For this review, take the finished solid that the model builds, in its own axes (mm). A direction names the side the tool comes from. Give positions to 0.01 mm unless a question says otherwise; leave off trailing zeros. Write each loop counter-clockwise with the first axis right and the second up, starting at its lowest first coordinate (ties: lowest second). Pieces come first, ordered by that corner, then holes.
Q1. Machinability: for faces 1 (the flat face through (-3.175, -3, -16)), 2 (the cylindrical face through (0.2, -3.1, 25.4)), which of the approach directions +Z, -Z, +X, -X, +Y, -Y give a long, thin tool a straight path to every point of the face, cutting with its end or side? Answer none if there is none.
Q2. We need section B-B (y = -1.5). Write out the cut boundary in (x, z) (3 decimals).
Q3. We need section C-C (z = -16.5). Write out the cut boundary in (x, y) (3 decimals), then the cut area to 3 significant figures.
Q4. Insertion check: P1, Ø3, axis at y = -4.5, z = -16.5, coming from the +X side; P2, Ø3, axis at y = -4.5, z = -16, coming from the -X side; P3, Ø1.5, axis at x = -21.5, y = -3.5, coming from the -Z side. Each pin has a flat end and moves straight along its axis. Give the tip position at first contact, or say it passes through.
Q5. Mouldability with a two-part tool opening along Z and no side actions: class faces 3 (the cylindrical face through (-19.212, -3.131, 11.173)), 4 (the flat face through (0, -3, -25.4)), 5 (the flat face through (-21.867, -3.131, 12.925)), 6 (the flat face through (7, -6.35, 2)) as released by +Z, released by -Z, zero draft, split by the parting line, or undercut.
Q6. We need section A-A (x = 0). Write out the cut boundary in (y, z) (3 decimals), then the cut area to 3 significant figures.
Q7. For line 1 (Z direction, x = 0, y = -2.5) (3 decimals); line 2 (X direction, y = -1.25, z = 9); line 3 (X direction, y = -4.5, z = 5), list the stretches that pass through material, from the lowest coordinate up.
Q8. We need section D-D (z = 0). Write out the cut boundary in (x, y), then the cut area to 3 significant figures.
```python
from build123d import *

# Parameters (mm, degrees)
F0_R     = 6.35
F1_DEPTH = 6.35
F3_DEPTH = 25.4


with BuildPart() as f1:
    # F0 (on Front) → F1 (new body)
    with BuildSketch(Plane.XZ):
        with BuildLine():
            Line((-18.594091, -25.4), (18.594091, -25.4))
            ThreePointArc((18.594091, -25.4), (21.997045, -12.7), (31.294091, -3.402955))
            Line((31.294091, -3.402955), (12.7, 28.802955))
            ThreePointArc((12.7, 28.802955), (0, 25.4), (-12.7, 28.802955))
            Line((-12.7, 28.802955), (-31.294091, -3.402955))
            ThreePointArc((-31.294091, -3.402955), (-21.997045, -12.7), (-18.594091, -25.4))
        make_face()
        Circle(F0_R, mode=Mode.SUBTRACT)
    extrude(amount=F1_DEPTH)

    # F2 (on Front) → F3 (cut)
    with BuildSketch(Plane.XZ):
        with BuildLine():
            Line((-3.175, -12.7), (-3.175, -19.05))
            ThreePointArc((-3.175, -19.05), (0, -22.225), (3.175, -19.05))
            Line((3.175, -19.05), (3.175, -12.7))
            ThreePointArc((3.175, -12.7), (0, -9.525), (-3.175, -12.7))
        make_face()
        with BuildLine():
            Line((-18.085284, 6.775369), (-12.586023, 3.600369))
            ThreePointArc((-12.586023, 3.600369), (-8.248892, 4.7625), (-9.411023, 9.099631))
            Line((-9.411023, 9.099631), (-14.910284, 12.274631))
            ThreePointArc((-14.910284, 12.274631), (-19.247415, 11.1125), (-18.085284, 6.775369))
        make_face()
        with BuildLine():
            Line((14.910284, 12.274631), (9.411023, 9.099631))
            ThreePointArc((9.411023, 9.099631), (8.248892, 4.7625), (12.586023, 3.600369))
            Line((12.586023, 3.600369), (18.085284, 6.775369))
            ThreePointArc((18.085284, 6.775369), (19.247415, 11.1125), (14.910284, 12.274631))
        make_face()
    extrude(amount=F3_DEPTH, mode=Mode.SUBTRACT)


solid = f1.part
```
Computed:
1. face 1: +Y, -Y
1. face 2: +Z, +Y, -Y
2. outline: (-31.294, -3.403) arc R25.4 cw to (-18.594, -25.4) - (18.594, -25.4) arc R25.4 cw to (31.294, -3.403) - (12.7, 28.803) arc R25.4 cw to (-12.7, 28.803) - close; hole (-18.085, 6.775) - (-12.586, 3.6) arc R3.175 ccw to (-9.411, 9.1) - (-14.91, 12.275) arc R3.175 ccw to start; hole circle Ø12.7 at (0, 0); hole (-3.175, -19.05) arc R3.175 ccw to (3.175, -19.05) - (3.175, -12.7) arc R3.175 ccw to (-3.175, -12.7) - close; hole (9.411, 9.1) arc R3.175 ccw to (12.586, 3.6) - (18.085, 6.775) arc R3.175 ccw to (14.91, 12.275) - close
3. outline: (-20.204, -6.35) - (-3.175, -6.35) - (-3.175, 0) - (-20.204, 0) - close; (3.175, -6.35) - (20.204, -6.35) - (20.204, 0) - (3.175, 0) - close
3. area: 216 mm2
4. P1: stops at x = 20.82
4. P2: stops at x = -21.05
4. P3: stops at z = -15.16
5. face 3: undercut
5. face 4: released by -Z
5. face 5: released by +Z
5. face 6: zero draft
6. outline: (-6.35, -25.4) - (0, -25.4) - (0, -22.225) - (-6.35, -22.225) - close; (-6.35, -9.525) - (0, -9.525) - (0, -6.35) - (-6.35, -6.35) - close; (-6.35, 6.35) - (0, 6.35) - (0, 25.4) - (-6.35, 25.4) - close
6. area: 161 mm2
7. line 1: z = -25.4 to -22.225, -9.525 to -6.35, 6.35 to 25.4
7. line 2: x = -24.13 to -19.63, -9.25 to 9.25, 19.63 to 24.13
7. line 3: x = -26.44 to -15.01, -8.12 to -3.91, 3.91 to 8.12, 15.01 to 26.44
8. outline: (-29.33, -6.35) - (-6.35, -6.35) - (-6.35, 0) - (-29.33, 0) - close; (6.35, -6.35) - (29.33, -6.35) - (29.33, 0) - (6.35, 0) - close
8. area: 292 mm2
